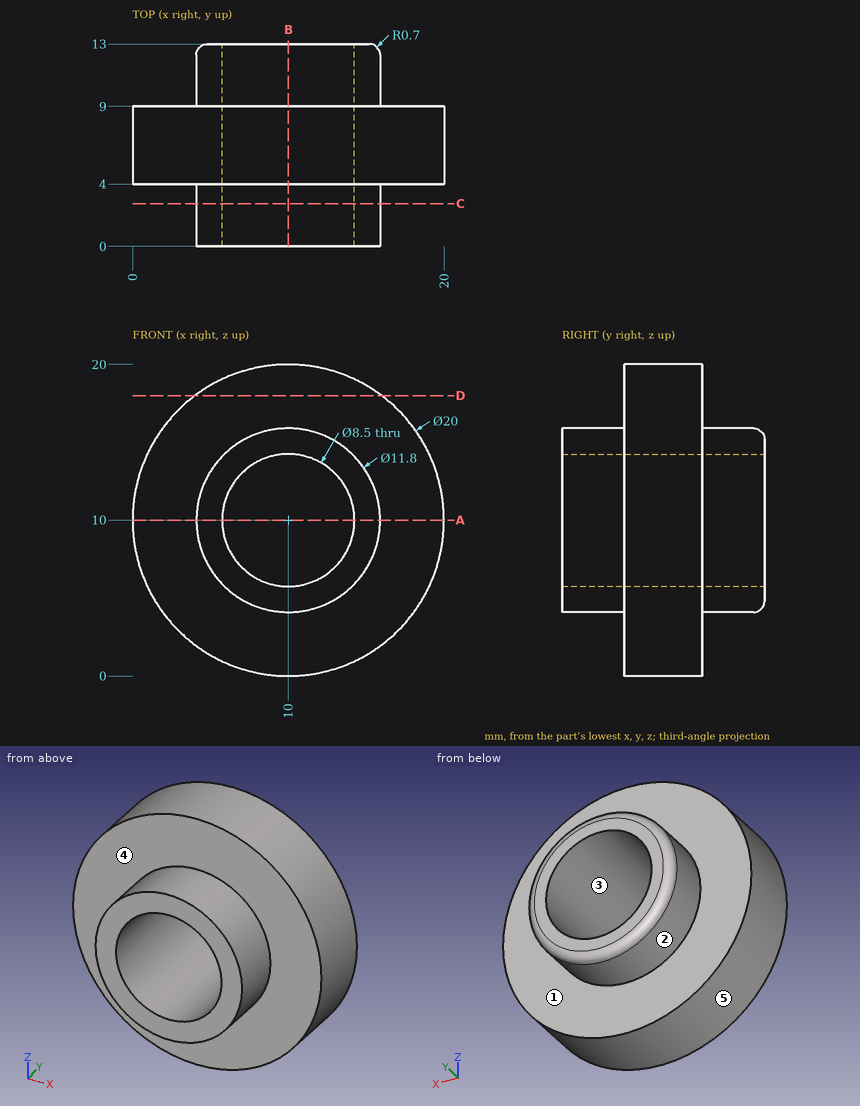
Part print with two shaded views. Sizes in mm from the minimum x, y, z corner. A direction names the side the tool comes from. Coordinates: 2 decimals unless noted, no trailing zeros. Write each loop counter-clockwise with the first axis right and the second up, starting at its lowest first coordinate (ties: lowest second). Pieces come first, ordered by that corner, then holes. Notation, with made-up numbers: (63, -6) - (105, -6) arc R13 cw to (105, 8) - close; hole circle Ø1 at (55.5, 67). An arc over 180 degrees is marked (long way). Put each result on its own line as item: value.
1. Two-plate mould, pull along X, no slides. Class the marked faces 1, 2 and 3: +X half, -X half, draft (parallel to the pull), parting line (faces both ways), or undercut.
Final values:
face 1: draft
face 2: parting line
face 3: undercut
2. Band-saw the part on B-B (x = 10). Write the cut outline in (y, z).
Final values:
outline: (0, 4.1) - (4, 4.1) - (4, 0) - (9, 0) - (9, 4.1) - (12.3, 4.1) arc R0.7 ccw to (13, 4.8) - (13, 5.75) - (0, 5.75) - close; (0, 14.25) - (13, 14.25) - (13, 15.2) arc R0.7 ccw to (12.3, 15.9) - (9, 15.9) - (9, 20) - (4, 20) - (4, 15.9) - (0, 15.9) - close
3. Probe line 1 along Z through (x, y) = (10, 8.25); line 2 along X through (y, z) = (8, 13.5); line 3 along Y through (x, z) = (1.75, 4.5). List the from-to ranges inside material, lowest first. Write a range as [from, to].
Final values:
line 1: z = [0, 5.75], [14.25, 20]
line 2: x = [0.63, 7.59], [12.41, 19.37]
line 3: y = [4, 9]
4. Band-saw the part on C-C (y = 2.75). Write the cut outline in (x, z).
Final values:
outline: circle Ø11.8 at (10, 10); hole circle Ø8.5 at (10, 10)
5. 3-axis set-ups, long thin cutter, end or side, ignore diameter. For the marked faces 4 and 5: which of +Z, -Z, +X, -X, +Y, -Y reach the whole face in a straight line?
Final values:
face 4: -Y
face 5: +Y, -Y
6. Band-saw the part on D-D (z = 18). Write the cut outline in (x, y).
Final values:
outline: (4, 4) - (16, 4) - (16, 9) - (4, 9) - close
7. Band-saw the part on A-A (z = 10). Write the cut outline in (x, y).
Final values:
outline: (0, 4) - (4.1, 4) - (4.1, 0) - (5.75, 0) - (5.75, 13) - (4.8, 13) arc R0.7 ccw to (4.1, 12.3) - (4.1, 9) - (0, 9) - close; (14.25, 0) - (15.9, 0) - (15.9, 4) - (20, 4) - (20, 9) - (15.9, 9) - (15.9, 12.3) arc R0.7 ccw to (15.2, 13) - (14.25, 13) - close
8. Flat gauge pins, fed straight in: pin 1 Ø2 at (x, y) = (3.5, 8) entering from +Z; pin 2 Ø3 at (y, z) = (4.5, 10.5) entering from -X; pin 3 Ø2 at (x, y) = (17.5, 10.5) entering from +Z; pin 4 Ø5 at (y, z) = (3.5, 3.5) entering from +X. Where does each tip first touch, or does it go through?
Final values:
pin 1: stops at z = 18.35
pin 2: stops at x = 0
pin 3: passes through
pin 4: stops at x = 19.14
